from build123d import *

# Parameters (mm, degrees)
SKETCH_1_W      = 35
SKETCH_1_H      = 3
EXTRUDE_1_DEPTH = 3


with BuildPart() as part:
    # Эскиз1 → Бобышка-Вытянуть1 (new body)
    with BuildSketch(Plane.XY):
        Polygon((14.215686275, 61.346405229), (76.715686275, 61.346405229), (76.715686275, 6.346405229), (-73.284313725, 6.346405229), (-73.284313725, 61.346405229), (-10.784313725, 61.346405229), (-10.784313725, 64.346405229), (14.215686275, 64.346405229), align=None)
        with Locations((1.715686275, 12.846405229)):
            Rectangle(SKETCH_1_W, SKETCH_1_H, mode=Mode.SUBTRACT)
    extrude(amount=EXTRUDE_1_DEPTH)


solid = part.part
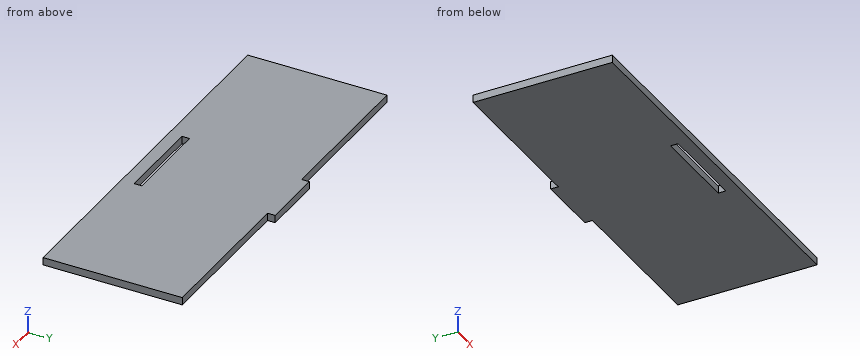
Geometry: final body of the model. Coordinates: model frame, mm. Round coordinates to 2 decimals unless told otherwise and drop trailing zeros. Loops run counter-clockwise (first coordinate to the right, second up) from the corner with the lowest first, then second, coordinate; pieces in that order, holes last.
Q1. Section A-A on x = 4. Return loops of the section in (y, z).
Q2. Section C-C on x = -24.5. Return loops of the section in (y, z), plus the area to 3 significant figures.
Q3. Material intervals for L1, parallel to Y at x = -3.5, z = 1.4; L2, parallel to X at y = 12, z = 2.4; L3, parallel to Y at x = 16, z = 2.65, sorted ascending.
Q4. Section B-B on z = 0.9. Return loops of the section in (x, y), plus the area to 3 significant figures.
Q5. Pin query (flat end, axial travel): P1, Ø12, axis at x = 30, y = 50, coming from the -Z side; P2, Ø0.9, axis at x = -49, z = 1.5, coming from the +Y side. Return the tip coordinate at first contact, or that it passes through.
Evaluation:
1. outline: (6.35, 0) - (11.35, 0) - (11.35, 3) - (6.35, 3) - close; (14.35, 0) - (64.35, 0) - (64.35, 3) - (14.35, 3) - close
2. outline: (6.35, 0) - (61.35, 0) - (61.35, 3) - (6.35, 3) - close
2. area: 165 mm2
3. L1: y = 6.35 to 11.35, 14.35 to 64.35
3. L2: x = -73.28 to -15.78, 19.22 to 76.72
3. L3: y = 6.35 to 11.35, 14.35 to 61.35
4. outline: (-73.28, 6.35) - (76.72, 6.35) - (76.72, 61.35) - (14.22, 61.35) - (14.22, 64.35) - (-10.78, 64.35) - (-10.78, 61.35) - (-73.28, 61.35) - close; hole (-15.78, 11.35) - (19.22, 11.35) - (19.22, 14.35) - (-15.78, 14.35) - close
4. area: 8,220 mm2
5. P1: stops at z = 0
5. P2: stops at y = 61.35
